Autodesk Inventor part; units mm, degrees
ref_plane "YZ Plane" through (0, 0, 0) normal (1, 0, 0) x (0, 1, 0)
ref_plane "XZ Plane" through (0, 0, 0) normal (0, 1, 0) x (-1, 0, 0)
ref_plane "XY Plane" through (0, 0, 0) normal (0, 0, 1) x (1, 0, 0)
sketch "Sketch1" plane through (0, 0, 0) normal (0, 1, 0) x (-1, 0, 0)
  circle A0 centre (0, 0) radius 4
  dimension "d7" = 8
extrude "Extrusion1" add sketch "Sketch1" along normal blind 1.5
sketch "Sketch2" plane through (0, 1.5, 0) normal (0, 1, 0) x (1, 0, 0)
  circle A0 centre (0, 0) radius 2.5
  dimension "d10" = 5
extrude "Extrusion2" add sketch "Sketch2" along normal blind 2
sketch "Sketch3" plane through (0, 3.5, 0) normal (0, 1, 0) x (1, 0, 0)
  circle A0 centre (0, 0) radius 2.5
  circle A1 centre (0, 0) radius 4
extrude "Extrusion3" add sketch "Sketch3" along normal blind 1.5 contours A0 | A1
sketch "Sketch5" plane through (0, 5, 0) normal (0, 1, 0) x (1, 0, 0)
  circle A0 centre (0, 0) radius 2.5
  circle A1 centre (0, 0) radius 4
  circle A2 centre (0, 0) radius 4
  line L0 (2, -3.4641) -> (-2, -3.4641)
  line L1 (-2, -3.4641) -> (-2, -8)
  line L2 (-2, -8) -> (2, -8)
  line L3 (2, -8) -> (2, -3.4641)
  dimension "d15" = 4
  dimension "d16" = 4
extrude "Extrusion4" add sketch "Sketch5" against normal blind 5 contours A1 L3 L2 L1
sketch "Sketch6" plane through (-2, 5, 8) normal (0, 0, 1) x (1, 0, 0)
  circle A0 centre (2, -2.5) radius 0.75
  line L0 (6, -1.5) -> (-2, -1.5)
  point P0 (2, -5)
  point P1 (4, -1.5)
  point P2 (0, -1.5)
  dimension "d21" = 1.5
  dimension "d27" = 1
extrude "Extrusion5" cut sketch "Sketch6" against normal blind 4.5
sketch "Sketch8" plane through (2, 5, 8) normal (1, 0, 0) x (0, 0, -1)
  line L0 (4.5359, -1.5) -> (4.5359, -3.5)
  line L1 (4.5359, -1.5) -> (4.5359, -3.5)
  line L2 (4.5359, -3.5) -> (2.5359, -3.5)
  line L3 (2.5359, -3.5) -> (2.5359, -1.5)
  line L4 (2.5359, -1.5) -> (4.5359, -1.5)
  point P0 (8, -5)
  dimension "d24" = 2
extrude "Extrusion6" cut sketch "Sketch8" against normal blind 4.5
fillet "Fillet1" radius 0.5 6 edges at (0, 3.5, 5.4641) (0, 1.5, 5.4641) (2, 4.25, 3.4641) (2, 0.75, 3.4641) (-2, 4.25, 3.4641) (-2, 0.75, 3.4641)
properties part number "Differential"
Part model, mm, in its own coordinate system. A direction names the side the tool comes from. Round coordinates to 2 decimals unless told otherwise and drop trailing zeros. Loops run counter-clockwise (first coordinate to the right, second up) from the corner with the lowest first, then second, coordinate; pieces in that order, holes last. Notation, with made-up numbers: (82, -8) -> (131, -8) arc R23 cw to (131, 29) -> close; hole circle Ø11 at (14.5, -26). An arc over 180 degrees is marked (long way). Use a Markdown table: item, result.
1) Cut at C-C, the plane x = 1.25. List the corners of the cut face in (y, z).
The answers:
| item | result |
|---|---|
| outline | (0, -3.8) -> (1.5, -3.8) -> (1.5, -2.17) -> (3.5, -2.17) -> (3.5, -3.8) -> (5, -3.8) -> (5, 8) -> (0, 8) -> close; hole (1.5, 2.17) -> (3.5, 2.17) -> (3.5, 4.96) arc R0.5 ccw to (3, 5.46) -> (2, 5.46) arc R0.5 ccw to (1.5, 4.96) -> close |
2) Tool access for faces 1 (the flat face through (2, 3, 6)), 2 (the flat face through (0, 1.5, 3)), 3 (the flat face through (1.3, 2.5, 5.464)): list every direction of +Z, -Z, +X, -X, +Y, -Y with a clear straight run to the whole face (end or side of a thin tool).
The answers:
| item | result |
|---|---|
| face 1 | +Z, +X, +Y, -Y |
| face 2 | none |
| face 3 | +X, -X |
3) Drop flat-ended pins along their axis: pin 1 Ø2 at (x, y) = (-2.5, 1.5) entering from -Z; pin 2 Ø2 at (y, z) = (3.5, 5.5) entering from +X; pin 3 Ø1.3 at (y, z) = (3.5, 5.5) entering from -X. Give the stop position or say it passes through.
The answers:
| item | result |
|---|---|
| pin 1 | stops at z = -3.71 |
| pin 2 | stops at x = 2 |
| pin 3 | stops at x = -2 |
4) Cut at A-A, the plane z = 4.75. List the corners of the cut face in (x, y).
The answers:
| item | result |
|---|---|
| outline | (-2, 0) -> (2, 0) -> (2, 1.5) -> (-2, 1.5) -> close; (-2, 3.5) -> (2, 3.5) -> (2, 5) -> (-2, 5) -> close |
5) Cut at B-B, the plane y = 2.2. List the corners of the cut face in (x, z), and give its area (3 significant figures).
The answers:
| item | result |
|---|---|
| outline | circle Ø5 at (0, 0); (-2, 5.46) -> (-0.69, 5.46) -> (-0.69, 8) -> (-2, 8) -> close; (0.69, 5.46) -> (2, 5.46) -> (2, 8) -> (0.69, 8) -> close |
| area | 26.3 mm2 |
6) Cut at D-D, the plane z = 0. List the corners of the cut face in (x, y), and give its area (3 significant figures).
The answers:
| item | result |
|---|---|
| outline | (-4, 0) -> (4, 0) -> (4, 1.5) -> (2.5, 1.5) -> (2.5, 3.5) -> (4, 3.5) -> (4, 5) -> (-4, 5) -> (-4, 3.5) -> (-2.5, 3.5) -> (-2.5, 1.5) -> (-4, 1.5) -> close |
| area | 34.0 mm2 |
7) Probe line 1 (X direction, y = 2.5, z = 6.2); line 2 (Y direction, x = 2.5, z = -1); line 3 (Y direction, x = 0, z = 6.7). List the from-to ranges inside material, lowest first. Write a range as [from, to].
The answers:
| item | result |
|---|---|
| line 1 | x = [-2, -0.75], [0.75, 2] |
| line 2 | y = [0, 1.5], [3.5, 5] |
| line 3 | y = [0, 1.75], [3.25, 5] |
8) Pull direction Z, two halves, no side cores. Call faces 4 (the cylindrical face through (-0.54, 2.49, -2.44)), 5 (the flat face through (0, 5, 2)), 6 (the flat face through (-1, 3, 8)): pulls with the +Z half, pulls with the -Z half, needs draft (parallel to the pull), parting line crosses it, or undercut.
The answers:
| item | result |
|---|---|
| face 4 | undercut |
| face 5 | needs draft |
| face 6 | pulls with the +Z half |
